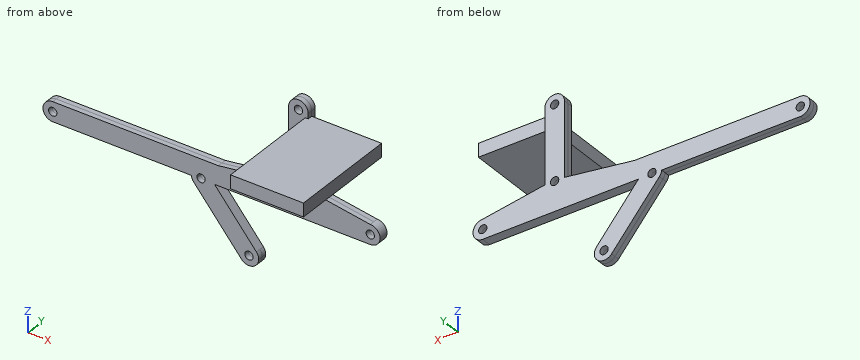
from build123d import *

# Parameters (mm, degrees)
F1_R     = 1.7
F2_DEPTH = 2
F3_W     = 29.8484290563
F3_H     = 5.5467073855
F4_DEPTH = 45


with BuildPart() as f2:
    # F1 (on Front) → F2 (new body, symmetric)
    with BuildSketch(Plane.XZ):
        with BuildLine():
            ThreePointArc((-41.5209898099, -12.0481280239), (-40.0251027901, -10.0182028071), (-38.1550220954, -11.7096733381))
            ThreePointArc((-38.1550220954, -11.7096733381), (-38.1635515644, -11.8797540328), (-38.189054381, -12.0481280239))
            Line((-38.189054381, -12.0481280239), (-35.8693667634, -12.0481280239))
            ThreePointArc((-35.8693667634, -12.0481280239), (-35.8586098715, -11.8790526048), (-35.8550220954, -11.7096733381))
            ThreePointArc((-35.8550220954, -11.7096733381), (-36.0962516123, -10.3415927648), (-36.790844323, -9.1385228994))
            ThreePointArc((-36.790844323, -9.1385228994), (-41.381040024, -8.0122053827), (-43.8406774275, -12.0481280239))
            Line((-43.8406774275, -12.0481280239), (-41.5209898099, -12.0481280239))
        make_face()
        with BuildLine():
            ThreePointArc((-38.189054381, -12.0481280239), (-39.8550220954, -13.4096733381), (-41.5209898099, -12.0481280239))
            Line((-41.5209898099, -12.0481280239), (-43.8406774275, -12.0481280239))
            ThreePointArc((-43.8406774275, -12.0481280239), (-43.5524900509, -13.2356912667), (-42.9191998679, -14.2808237769))
            ThreePointArc((-42.9191998679, -14.2808237769), (-38.6473330608, -15.5230035357), (-35.8693667634, -12.0481280239))
            Line((-35.8693667634, -12.0481280239), (-38.189054381, -12.0481280239))
        make_face()
        with BuildLine():
            Line((-100.580998737, -12.0481280239), (-43.8406774275, -12.0481280239))
            ThreePointArc((-43.8406774275, -12.0481280239), (-41.381040024, -8.0122053827), (-36.790844323, -9.1385228994))
            Line((-36.790844323, -9.1385228994), (-34.3493957361, -12.0481280239))
            Line((-34.3493957361, -12.0481280239), (29.419001263, -12.0481280239))
            ThreePointArc((29.419001263, -12.0481280239), (25.419001263, -8.0481280239), (29.419001263, -4.0481280239))
            Line((29.419001263, -4.0481280239), (-32.7925062924, -4.0481280239))
            Line((-32.7925062924, -4.0481280239), (-100.580998737, -4.0481280239))
            ThreePointArc((-100.580998737, -4.0481280239), (-97.7525716123, -5.2197008992), (-96.580998737, -8.0481280239))
            ThreePointArc((-96.580998737, -8.0481280239), (-97.7525716123, -10.8765551487), (-100.580998737, -12.0481280239))
        make_face()
        with BuildLine():
            ThreePointArc((-35.8550220954, -11.7096733381), (-35.8586098715, -11.8790526048), (-35.8693667634, -12.0481280239))
            Line((-35.8693667634, -12.0481280239), (-34.3493957361, -12.0481280239))
            Line((-34.3493957361, -12.0481280239), (-36.790844323, -9.1385228994))
            ThreePointArc((-36.790844323, -9.1385228994), (-36.0962516123, -10.3415927648), (-35.8550220954, -11.7096733381))
        make_face()
        with BuildLine():
            Line((-34.3493957361, -12.0481280239), (-35.8693667634, -12.0481280239))
            ThreePointArc((-35.8693667634, -12.0481280239), (-38.6473330608, -15.5230035357), (-42.9191998679, -14.2808237769))
            Line((-42.9191998679, -14.2808237769), (-23.3141777725, -37.645179292))
            ThreePointArc((-23.3141777725, -37.645179292), (-22.8211504387, -32.0098510808), (-17.1858222275, -32.5028784145))
            Line((-17.1858222275, -32.5028784145), (-34.3493957361, -12.0481280239))
        make_face()
        with BuildLine():
            ThreePointArc((-100.580998737, -4.0481280239), (-104.580998737, -8.0481280239), (-100.580998737, -12.0481280239))
            ThreePointArc((-100.580998737, -12.0481280239), (-97.7525716123, -10.8765551487), (-96.580998737, -8.0481280239))
            ThreePointArc((-96.580998737, -8.0481280239), (-97.7525716123, -5.2197008992), (-100.580998737, -4.0481280239))
        make_face()
        with Locations((-100.580998737, -8.0481280239)):
            Circle(F1_R, mode=Mode.SUBTRACT)
        with BuildLine():
            ThreePointArc((-17.1858222275, -32.5028784145), (-22.8211504387, -32.0098510808), (-23.3141777725, -37.645179292))
            ThreePointArc((-23.3141777725, -37.645179292), (-18.8819194267, -38.8327993364), (-16.25, -35.0740288533))
            ThreePointArc((-16.25, -35.0740288533), (-16.4912295169, -33.70594828), (-17.1858222275, -32.5028784145))
        make_face()
        with Locations((-20.25, -35.0740288533)):
            Circle(F1_R, mode=Mode.SUBTRACT)
        with BuildLine():
            ThreePointArc((29.419001263, -4.0481280239), (25.419001263, -8.0481280239), (29.419001263, -12.0481280239))
            ThreePointArc((29.419001263, -12.0481280239), (32.2474283877, -10.8765551487), (33.419001263, -8.0481280239))
            ThreePointArc((33.419001263, -8.0481280239), (32.2474283877, -5.2197008992), (29.419001263, -4.0481280239))
        make_face()
        with Locations((29.419001263, -8.0481280239)):
            Circle(F1_R, mode=Mode.SUBTRACT)
        with BuildLine():
            Line((-4, 0), (-32.7925062924, -4.0481280239))
            Line((-32.7925062924, -4.0481280239), (29.419001263, -4.0481280239))
            Line((29.419001263, -4.0481280239), (4, 0))
            ThreePointArc((4, 0), (0, -4), (-4, 0))
        make_face()
        with BuildLine():
            Line((-4, 30.5), (-4, 0))
            ThreePointArc((-4, 0), (0, 4), (4, 0))
            Line((4, 0), (4, 30.5))
            ThreePointArc((4, 30.5), (0, 26.5), (-4, 30.5))
        make_face()
        with BuildLine():
            ThreePointArc((4, 0), (0, 4), (-4, 0))
            ThreePointArc((-4, 0), (0, -4), (4, 0))
        make_face()
        Circle(F1_R, mode=Mode.SUBTRACT)
        with BuildLine():
            ThreePointArc((4, 30.5), (0, 34.5), (-4, 30.5))
            ThreePointArc((-4, 30.5), (0, 26.5), (4, 30.5))
        make_face()
        with Locations((0, 30.5)):
            Circle(F1_R, mode=Mode.SUBTRACT)
    extrude(amount=F2_DEPTH, both=True)

    # F3 (on Front) → F4 (join)
    with BuildSketch(Plane.XZ):
        with Locations((17.7185675129, 25.5892256688)):
            Rectangle(F3_W, F3_H)
    extrude(amount=F4_DEPTH)


solid = f2.part
For this review, take the finished solid that the model builds, in its own axes (mm). Round coordinates to 2 decimals unless told otherwise and drop trailing zeros. Order: outer loops, then holes, each group sorted by start corner. A loop starts at its lowest first (then second) coordinate and runs counter-clockwise, first axis right, second up. Notation, with made-up numbers: M -31,15 L 2,15 A24 ccw 2,28 Z; hole C -16.75,80.5 d8. An arc over 180 degrees is marked long. Use a Markdown table: item, result. Add a question column.
Item 1: To check wall thickness, follow line 1 along Z through (x, y) = (0, 1.1); line 2 along Z through (x, y) = (-20.5, 0.5); line 3 along Z through (x, y) = (7, -5). State the ranges of each line that lie inside material, in increasing order.
Item 2: Insertion check: pin 1 (3 mm diameter, centred on x = -20.25, z = -35.07, fed in from +Y); pin 2 (24 mm diameter, centred on x = 14.5, y = -16, fed in from +Z); pin 3 (0.6 mm diameter, centred on y = -0.5, z = 14, fed in from -X); pin 4 (6 mm diameter, centred on x = -78.5, z = -12.5, fed in from -Y). Each pin has a flat end and moves straight along its axis. Give the tip position at first contact, or say it passes through.
Item 3: Add section A-A, the plane x = 0. Give the boundary of the cut face in (y, z), then the cut area to 3 significant figures.
Item 4: Add section C-C, the plane x = -20.25. Give the boundary of the cut face in (y, z).
Item 5: Add section D-D, the plane y = -10. Give the boundary of the cut face in (x, z), then the cut area to 3 significant figures.
Item 6: Add section B-B, the plane z = 25. Give the boundary of the cut face in (x, y), then the cut area to 3 significant figures.
Geometry results:
| question | item | result |
|---|---|---|
| 1 | line 1 | z = -12.05 to -1.7, 1.7 to 28.8, 32.2 to 34.5 |
| 1 | line 2 | z = -39.07 to -36.76, -33.39 to -28.55, -12.05 to -2.32 |
| 1 | line 3 | z = 22.82 to 28.36 |
| 2 | pin 1 | passes through |
| 2 | pin 2 | stops at z = 28.36 |
| 2 | pin 3 | stops at x = -4 |
| 2 | pin 4 | stops at y = -2 |
| 3 | outline | M -2,-12.05 L 2,-12.05 L 2,-1.7 L -2,-1.7 Z; M -2,1.7 L 2,1.7 L 2,28.8 L -2,28.8 Z; M -2,32.2 L 2,32.2 L 2,34.5 L -2,34.5 Z |
| 3 | area | 159 mm² |
| 4 | outline | M -2,-39.07 L 2,-39.07 L 2,-36.77 L -2,-36.77 Z; M -2,-33.37 L 2,-33.37 L 2,-28.85 L -2,-28.85 Z; M -2,-12.05 L 2,-12.05 L 2,-2.28 L -2,-2.28 Z |
| 5 | outline | M 2.79,22.82 L 32.64,22.82 L 32.64,28.36 L 2.79,28.36 Z |
| 5 | area | 166 mm² |
| 6 | outline | M -4,-2 L 2.79,-2 L 2.79,-45 L 32.64,-45 L 32.64,0 L 4,0 L 4,2 L -4,2 Z |
| 6 | area | 1,370 mm² |
